Can you work these out from the model? Positions are in its coordinate system, mm. A direction names the side the tool comes from. Coordinates: 2 decimals unless noted, no trailing zeros. Loops run counter-clockwise (first coordinate to the right, second up) from the corner with the lowest first, then second, coordinate; pieces in that order, holes last. Notation, with made-up numbers: M 46,31.5 L 84,31.5 A17 cw 84,47.5 Z; hole C 58.5,2 d2. An arc over 180 degrees is marked long. Answer as a JSON object with one key per item and string values. Group by question number.
Item 1: If I drill on line 1 (Y direction, x = 0, z = 15); line 2 (X direction, y = -14, z = 5); line 3 (X direction, y = 1.5, z = 21.25), over which ranges is the centre line in solid material (lowest first)?
Item 2: Suppose I cut it at A-A (y = 0). Write out the boundary of the cut face in (x, z).
Item 3: Which directions (+Z, -Z, +X, -X, +Y, -Y) give clear straight access to the entire face, cutting with the end or side of a thin tool? Please do faces 1 (the flat face through (-14, -1.75, 3)), 2 (the flat face through (-1.75, -14, 3)), 3 (the flat face through (1.75, 14, 3)), 4 (the cylindrical face through (-6.269, 4.807, 16.32)).
Item 4: We'd pull the mould along Y, two halves only. Please class faces 5 (the flat face through (-7, 4, 6.46)), 6 (the cylindrical face through (-0.878, 3.954, 13.045)), 7 (the cylindrical face through (-11.242, 11.031, 3.185)), 8 (the cylindrical face through (-10.403, 0.038, 3.185)): +Y half, -Y half, draft (parallel to the pull), parting line (faces both ways), or undercut.
Item 5: I'm going to push flat-ended pins straight in: pin 1 Ø4 at (y, z) = (14.5, 3) entering from -X; pin 2 Ø1.8 at (x, z) = (-13.5, 2.5) entering from -Y; pin 3 Ø1 at (y, z) = (13.5, 2) entering from +X. Where does each tip first touch, or does it pass through?
Item 6: Suppose I cut it at D-D (y = 6). Write out the boundary of the cut face in (x, z), then the cut area to 3 significant figures.
Item 7: Suppose I cut it at C-C (z = 2.25). Write out the boundary of the cut face in (x, y).
Autodesk Inventor part; units mm, degrees
ref_plane "YZ Plane" through (0, 0, 0) normal (1, 0, 0) x (0, 1, 0)
ref_plane "XZ Plane" through (0, 0, 0) normal (0, 1, 0) x (-1, 0, 0)
ref_plane "XY Plane" through (0, 0, 0) normal (0, 0, 1) x (1, 0, 0)
sketch "Sketch1" plane through (0, 0, 0) normal (0, 0, 1) x (1, 0, 0)
  circle A0 centre (0, 0) radius 15.75
  circle A1 centre (0, 0) radius 4.05
  dimension "d0" = 31.5
  dimension "d1" = 8.1
extrude "Extrusion1" add sketch "Sketch1" along normal blind 6.46
sketch "Sketch2" plane through (0, 0, 6.46) normal (0, 0, 1) x (1, 0, 0)
  circle A0 centre (0, 0) radius 4.05
  circle A1 centre (0, 0) radius 15.75
  circle A2 centre (0, 0) radius 7.9
  circle A3 centre (0, 0) radius 4.05
  dimension "d4" = 15.8
extrude "Extrusion2" add sketch "Sketch2" along normal blind 20 contours A2
sketch "Sketch3" plane through (0, 0, 0) normal (0, 0, -1) x (-1, 0, 0)
  circle A0 centre (0, 0) radius 4.05
  circle A1 centre (0, 0) radius 15.75
  line L0 (-1.75, 15.6525) -> (-1.75, 12.1525)
  line L1 (1.75, 12.1525) -> (1.75, 15.6525)
  arc A2 (-1.75, 12.1525) -> (1.75, 12.1525) centre (0, 12.1525) ccw
  arc A3 (1.75, 15.6525) -> (-1.75, 15.6525) centre (0, 0) ccw
  dimension "d7" = 3.5
  dimension "d8" = 3.5
extrude "Extrusion3" cut sketch "Sketch3" against normal blind 20 contours L1 A2 L0 A1 picked at (0.1948, 13.3481)
pattern_circular "Circular Pattern1" count 4 over 360 about axis through (0, 0, 0) along (0, 0, 1) of "Extrusion3"
properties part number "Nut"
From the geometry:
{
 "1": {"line 1": "-7.9 to -4.05, 4.05 to 7.9", "line 2": "-7.22 to -1.75, 1.75 to 7.22", "line 3": "-7.76 to -3.76, 3.76 to 7.76"},
 "2": {"outline": "M -10.4,0 L -4.05,0 L -4.05,26.46 L -7.9,26.46 L -7.9,6.46 L -10.4,6.46 Z; M 4.05,0 L 10.4,0 L 10.4,6.46 L 7.9,6.46 L 7.9,26.46 L 4.05,26.46 Z"},
 "3": {"face 1": "+Z, -Z, -X", "face 2": "+Z, -Z, -Y", "face 3": "+Z, -Z, +Y", "face 4": "+Z"},
 "4": {"face 5": "draft", "face 6": "undercut", "face 7": "+Y half", "face 8": "undercut"},
 "5": {"pin 1": "x = -9.58", "pin 2": "y = -9.45", "pin 3": "x = 8.89"},
 "6": {"outline": "M -14.56,0 L 14.56,0 L 14.56,6.46 L 5.14,6.46 L 5.14,26.46 L -5.14,26.46 L -5.14,6.46 L -14.56,6.46 Z", "area": "394 mm2"},
 "7": {"outline": "M -15.65,-1.75 A15.75 ccw -1.75,-15.65 L -1.75,-12.15 A1.75 cw 1.75,-12.15 L 1.75,-15.65 A15.75 ccw 15.65,-1.75 L 12.15,-1.75 A1.75 cw 12.15,1.75 L 15.65,1.75 A15.75 ccw 1.75,15.65 L 1.75,12.15 A1.75 cw -1.75,12.15 L -1.75,15.65 A15.75 ccw -15.65,1.75 L -12.15,1.75 A1.75 cw -12.15,-1.75 Z; hole C 0,0 d8.1"}
}
